Geometry: final body of the model. Coordinates: model frame, mm. A direction names the side the tool comes from. Give positions to 0.01 mm unless a question says otherwise; leave off trailing zeros. Write each loop counter-clockwise with the first axis right and the second up, starting at its lowest first coordinate (ties: lowest second). Pieces come first, ordered by that corner, then holes.
from build123d import *

# Parameters (mm, degrees)
EXTRUDE_1_DEPTH        = 8
HOLE_WIZARD_M4_1_D     = 3.3
CUT_EXTRUDE_1_DEPTH    = 3.5
CUT_EXTRUDE_2_DEPTH    = 62.613716005
PATTERN_LINEAR_1_COUNT = 2
PATTERN_LINEAR_1_PITCH = 12
CHAMFER_1_SIZE         = 1
CHAMFER_2_SIZE         = 0.5
PATTERN_LINEAR_2_COUNT = 2
PATTERN_LINEAR_2_PITCH = 20


with BuildPart() as part:
    # 草图1 → 凸台-拉伸1 (new body)
    with BuildSketch(Plane.XY):
        Polygon((0, 0), (-32, 0), (-32, 11), (-60, 11), (-60, 15), (0, 15), align=None)
    extrude(amount=EXTRUDE_1_DEPTH)

    # M4 螺纹孔1 (through all)
    with Locations(Plane(origin=(0, 15, 0), x_dir=(-1, 0, 0), z_dir=(0, 1, 0))):
        with Locations((56, 4)):
            hole_wizard_m4_1 = Hole(HOLE_WIZARD_M4_1_D / 2)

    # 草图4 → 切除-拉伸1 (cut)
    with BuildSketch(Plane(origin=(0, 15, 0), x_dir=(1, 0, 0), z_dir=(0, 1, 0))):
        with BuildLine():
            Line((-15.75, -7), (-20.25, -7))
            ThreePointArc((-20.25, -7), (-23.25, -4), (-20.25, -1))
            Line((-20.25, -1), (-15.75, -1))
            ThreePointArc((-15.75, -1), (-12.75, -4), (-15.75, -7))
        make_face()
    cut_extrude_1 = extrude(amount=-CUT_EXTRUDE_1_DEPTH, mode=Mode.SUBTRACT)

    # 草图5 → 切除-拉伸2 (cut, through all)
    with BuildSketch(Plane(origin=(0, 11.5, 0), x_dir=(1, 0, 0), z_dir=(0, 1, 0))):
        with BuildLine():
            Line((-20.25, -5.75), (-15.75, -5.75))
            ThreePointArc((-15.75, -5.75), (-14, -4), (-15.75, -2.25))
            Line((-15.75, -2.25), (-20.25, -2.25))
            ThreePointArc((-20.25, -2.25), (-22, -4), (-20.25, -5.75))
        make_face()
    cut_extrude_2 = extrude(amount=-CUT_EXTRUDE_2_DEPTH, mode=Mode.SUBTRACT)

    # 阵列(线性)1: 切除-拉伸1, 切除-拉伸2 ×2
    with Locations(*[(i * PATTERN_LINEAR_1_PITCH, 0, 0) for i in range(1, PATTERN_LINEAR_1_COUNT)]):
        add(cut_extrude_1, mode=Mode.SUBTRACT)
        add(cut_extrude_2, mode=Mode.SUBTRACT)

    # 倒角1
    chamfer_1_edges = [part.edges().sort_by_distance(p)[0] for p in [
        (-60, 13, 8),
        (-60, 13, 0),
    ]]
    chamfer(chamfer_1_edges, length=CHAMFER_1_SIZE)

    # 倒角2
    chamfer_2_edges = [part.edges().sort_by_distance(p)[0] for p in [
        (0, 0, 4),
        (-32, 5.5, 8),
        (-16, 0, 8),
        (0, 7.5, 8),
        (-32, 5.5, 0),
        (-16, 0, 0),
        (0, 7.5, 0),
        (-29.5, 15, 0),
        (0, 15, 4),
        (-29.5, 15, 8),
        (-60, 11, 4),
        (-60, 15, 4),
        (-45.5, 11, 8),
        (-32, 0, 4),
        (-45.5, 11, 0),
    ]]
    chamfer(chamfer_2_edges, length=CHAMFER_2_SIZE - 0.0001)  # a hair under: the kernel refuses the full size

    # 阵列(线性)2: M4 螺纹孔1 ×2
    with Locations(*[(i * PATTERN_LINEAR_2_PITCH, 0, 0) for i in range(1, PATTERN_LINEAR_2_COUNT)]):
        add(hole_wizard_m4_1, mode=Mode.SUBTRACT)


solid = part.part
Q1. Section A-A on x = -56. Output: boundary loops of the cut face in (y, z).
Filled sheet:
outline: (11, 0.5) - (11.5, 0) - (14.5, 0) - (15, 0.5) - (15, 2.35) - (11, 2.35) - close; (11, 5.65) - (15, 5.65) - (15, 7.5) - (14.5, 8) - (11.5, 8) - (11, 7.5) - close
Q2. Section D-D on z = 4. Count the separate pieces of the cut face and the enclosed holes in it, plus the area to 3 significant figures.
Filled sheet:
separate pieces: 5
enclosed holes: 0
area: 307 mm2
Q3. Section C-C on x = -45.5. Output: boundary loops of the cut face in (y, z), plus the area to 3 significant figures.
Filled sheet:
outline: (11, 0.5) - (11.5, 0) - (14.5, 0) - (15, 0.5) - (15, 7.5) - (14.5, 8) - (11.5, 8) - (11, 7.5) - close
area: 31.5 mm2
Q4. Ray query, line 1 along Z through (x, y) = (-19.5, 4.5); line 2 along Z through (x, y) = (-56, 14.05); line 3 along X through (y, z) = (1.5, 3). Return the intervals inside material, ascending.
Filled sheet:
line 1: z = 0 to 2.25, 5.75 to 8
line 2: z = 0 to 2.35, 5.65 to 8
line 3: x = -32 to -21.69, -14.31 to -9.69, -2.31 to 0
Q5. Pin query (flat end, axial travel): P1, Ø4.5, axis at x = -36, z = 4, coming from the -Y side; P2, Ø1.8, axis at x = -19.5, z = 5, coming from the +Y side. Return the tip coordinate at first contact, or that it passes through.
Filled sheet:
P1: stops at y = 11
P2: stops at y = 11.5
Q6. Section B-B on y = 8. Output: boundary loops of the cut face in (x, z).
Filled sheet:
outline: (-32, 0.5) - (-31.5, 0) - (-0.5, 0) - (0, 0.5) - (0, 7.5) - (-0.5, 8) - (-31.5, 8) - (-32, 7.5) - close; hole (-20.25, 2.25) - (-15.75, 2.25) arc R1.75 ccw to (-15.75, 5.75) - (-20.25, 5.75) arc R1.75 ccw to start; hole (-8.25, 2.25) - (-3.75, 2.25) arc R1.75 ccw to (-3.75, 5.75) - (-8.25, 5.75) arc R1.75 ccw to start
Q7. Access query for faces 4 (the flat face through (-32, 6, 4)), 5 (the flat face through (-60, 13, 4)), 6 (the cylindrical face through (-2, 6, 4)), 7 (the cylindrical face through (-0.75, 13.27, 3.93)), 8 (the flat face through (-23, 9, 8)). Directions: +Z, -Z, +X, -X, +Y, -Y. A direction counts if a zero-diameter tool reaches every point of the face in a straight line with its end or side. Return the directions, or none.
Filled sheet:
face 4: +Z, -Z, -X, -Y
face 5: +Z, -Z, -X, +Y, -Y
face 6: +Y, -Y
face 7: +Y
face 8: +Z, +X, -X, +Y, -Y
Q8. Pull-direction query (Z, two-part tool) for faces 1 (the cylindrical face through (-11.25, 13.27, 4.07)), 2 (the flat face through (0, 8, 4)), 3 (the flat face through (-59.5, 13, 7.5)); classes: released by +Z, released by -Z, zero draft, split by the parting line, or undercut.
Filled sheet:
face 1: undercut
face 2: zero draft
face 3: released by +Z
